Could you check a few things on this model? Use its own coordinates, in mm. Face numbers are marked on the shaded views. A direction names the side the tool comes from. Give positions to 0.01 mm unless a question says otherwise; leave off trailing zeros. Loops run counter-clockwise (first coordinate to the right, second up) from the corner with the lowest first, then second, coordinate; pieces in that order, holes last. Notation, with made-up numbers: (13.5, 50) -> (26.5, 50) arc R12 ccw to (26.5, 70) -> close; hole circle Ø1 at (55.25, 53). An arc over 180 degrees is marked (long way). Put each result on its own line as item: value.
```python
from build123d import *

# Parameters (mm, degrees)
SKETCH1_R           = 1.5
BOSS_EXTRUDE1_DEPTH = 0.85
SKETCH2_W           = 4.5
SKETCH2_H           = 18.4
BOSS_EXTRUDE2_DEPTH = 3
SKETCH3_W           = 6
SKETCH3_H           = 4.5
BOSS_EXTRUDE3_DEPTH = 3
SKETCH4_W           = 7.5
SKETCH4_H           = 5.75
BOSS_EXTRUDE4_DEPTH = 2.3
SKETCH5_W           = 20.5
SKETCH5_H           = 15.8
BOSS_EXTRUDE5_DEPTH = 7.65
SKETCH6_W           = 2.5
SKETCH6_H           = 5
BOSS_EXTRUDE6_DEPTH = 8.6
SKETCH7_W           = 20.5
SKETCH7_H           = 7
BOSS_EXTRUDE7_DEPTH = 2


with BuildPart() as part:
    # Sketch1 → Boss-Extrude1 (new, symmetric)
    with BuildSketch(Plane(origin=(0, 0, 0), x_dir=(1, 0, 0), z_dir=(0, 1, 0))):
        with BuildLine():
            Line((-15, -18), (15, -18))
            ThreePointArc((15, -18), (17.121320344, -17.121320344), (18, -15))
            Line((18, -15), (18, 15))
            ThreePointArc((18, 15), (17.121320344, 17.121320344), (15, 18))
            Line((15, 18), (-15, 18))
            ThreePointArc((-15, 18), (-17.121320344, 17.121320344), (-18, 15))
            Line((-18, 15), (-18, -15))
            ThreePointArc((-18, -15), (-17.121320344, -17.121320344), (-15, -18))
        make_face()
        with Locations(Location((-15.25, 15.25, 0), (0, 0, 270))):
            Circle(SKETCH1_R, mode=Mode.SUBTRACT)
        with Locations(Location((15.25, 15.25, 0), (0, 0, 90))):
            Circle(SKETCH1_R, mode=Mode.SUBTRACT)
        with Locations(Location((15.25, -15.25, 0), (0, 0, 270))):
            Circle(SKETCH1_R, mode=Mode.SUBTRACT)
        with Locations(Location((-15.25, -15.25, 0), (0, 0, 90))):
            Circle(SKETCH1_R, mode=Mode.SUBTRACT)
    extrude(amount=BOSS_EXTRUDE1_DEPTH, both=True)

    # Sketch2 → Boss-Extrude2 (add)
    with BuildSketch(Plane(origin=(0, 0.85, 0), x_dir=(1, 0, 0), z_dir=(0, 1, 0))):
        with Locations((-15.75, -2.4)):
            Rectangle(SKETCH2_W, SKETCH2_H)
        with Locations((15.75, -2.4)):
            Rectangle(SKETCH2_W, SKETCH2_H)
    extrude(amount=BOSS_EXTRUDE2_DEPTH)

    # Sketch3 → Boss-Extrude3 (add)
    with BuildSketch(Plane(origin=(0, 0.85, 0), x_dir=(1, 0, 0), z_dir=(0, 1, 0))):
        with Locations((-9, 15.75)):
            Rectangle(SKETCH3_W, SKETCH3_H)
        with Locations((9, 15.75)):
            Rectangle(SKETCH3_W, SKETCH3_H)
    boss_extrude3 = extrude(amount=BOSS_EXTRUDE3_DEPTH)

    # Mirror2: Boss-Extrude3 across plane
    add(boss_extrude3.mirror(Plane.ZX))

    # Sketch4 → Boss-Extrude4 (add)
    with BuildSketch(Plane(origin=(0, 0.85, 0), x_dir=(1, 0, 0), z_dir=(0, 1, 0))):
        with Locations((0, 15.525)):
            Rectangle(SKETCH4_W, SKETCH4_H)
    extrude(amount=BOSS_EXTRUDE4_DEPTH)

    # Sketch5 → Boss-Extrude5 (add)
    with BuildSketch(Plane(origin=(0, 0.85, 0), x_dir=(1, 0, 0), z_dir=(0, 1, 0))):
        with Locations((-0.95, -19.15)):
            Rectangle(SKETCH5_W, SKETCH5_H)
    extrude(amount=BOSS_EXTRUDE5_DEPTH)

    # Sketch6 → Boss-Extrude6 (add)
    with BuildSketch(Plane(origin=(0, 0.85, 0), x_dir=(1, 0, 0), z_dir=(0, 1, 0))):
        with Locations((11.3, -15.5)):
            Rectangle(SKETCH6_W, SKETCH6_H)
    extrude(amount=BOSS_EXTRUDE6_DEPTH)

    # Sketch7 → Boss-Extrude7 (add)
    with BuildSketch(Plane.XZ.offset(0.85)):
        with Locations((-0.95, 14.5)):
            Rectangle(SKETCH7_W, SKETCH7_H)
    extrude(amount=BOSS_EXTRUDE7_DEPTH)


solid = part.part
```
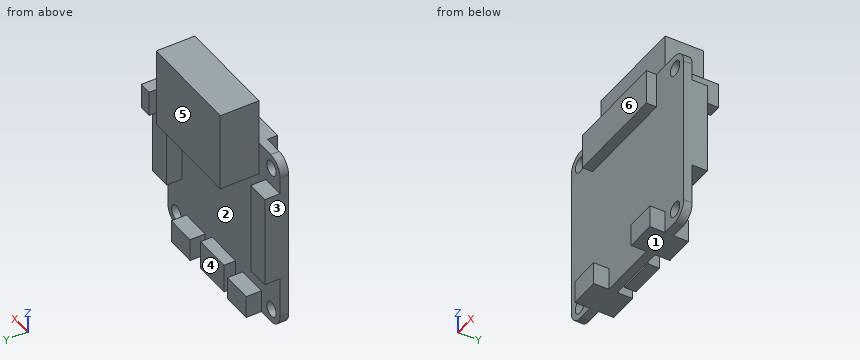
1. If we section it at A-A (y = 6.75): List the corners of the cut face in (x, z) for me.
Recorded:
outline: (-11.2, 11.25) -> (9.3, 11.25) -> (9.3, 27.05) -> (-11.2, 27.05) -> close; (10.05, 13) -> (12.55, 13) -> (12.55, 18) -> (10.05, 18) -> close
2. I need wall thicknesses on line 1 (X direction, y = 0.2, z = -15.25); line 2 (Z direction, x = 3, y = 2.25); line 3 (Z direction, x = 16, y = 0.75). Which ranges of each line are inside material? Lowest first, please.
Recorded:
line 1: x = -17.99 to -16.75, -13.75 to 13.75, 16.75 to 17.99
line 2: z = -18.4 to -12.65, 11.25 to 27.05
line 3: z = -17.83 to -16.55, -13.95 to 13.95, 16.55 to 17.83
3. If we section it at D-D (z = 12.5): List the corners of the cut face in (x, y) for me.
Recorded:
outline: (-18, -0.85) -> (-11.2, -0.85) -> (-11.2, -2.85) -> (9.3, -2.85) -> (9.3, -0.85) -> (18, -0.85) -> (18, 0.85) -> (9.3, 0.85) -> (9.3, 8.5) -> (-11.2, 8.5) -> (-11.2, 0.85) -> (-18, 0.85) -> close
4. Thinking about a two-plate mould opening in X: for the marked faces 1, 2 and 3, which applies, pulls with the +X half, pulls with the -X half, needs draft (parallel to the pull), parting line crosses it, or undercut?
Recorded:
face 1: needs draft
face 2: undercut
face 3: pulls with the -X half
5. If we section it at C-C (y = -2.25): List the corners of the cut face in (x, z) for me, then the cut area to 4 significant figures.
Recorded:
outline: (-12, -18) -> (-6, -18) -> (-6, -13.5) -> (-12, -13.5) -> close; (-11.2, 11) -> (9.3, 11) -> (9.3, 18) -> (-11.2, 18) -> close; (6, -18) -> (12, -18) -> (12, -13.5) -> (6, -13.5) -> close
area: 197.5 mm^2
6. I'm going to push flat-ended pins straight in: pin 1 (3 mm diameter, centred on x = -14, z = -1, fed in from -Y); pin 2 (3 mm diameter, centred on y = 6, z = 3.5, fed in from +X); pin 3 (3 mm diameter, centred on x = 6.5, y = 4.5, fed in from -Z); pin 4 (1.5 mm diameter, centred on y = 1.5, z = -16, fed in from -X). Where does each tip first touch, or does it pass through?
Recorded:
pin 1: stops at y = -0.85
pin 2: passes through
pin 3: stops at z = -18
pin 4: stops at x = -17.93
7. For the marked faces 4, 5 and 6, which set-ups out of +Z, -Z, +X, -X, +Y, -Y let a thin tool reach every point of the face, with its end or its side?
Recorded:
face 4: -Z, +Y
face 5: +Z, -Z, -X, +Y
face 6: +Z, +X, -X, -Y
8. If we section it at B-B (x = -6.5): List the corners of the cut face in (y, z) for me.
Recorded:
outline: (-3.85, -18) -> (3.85, -18) -> (3.85, -13.5) -> (0.85, -13.5) -> (0.85, 11.25) -> (8.5, 11.25) -> (8.5, 27.05) -> (0.85, 27.05) -> (0.85, 18) -> (-2.85, 18) -> (-2.85, 11) -> (-0.85, 11) -> (-0.85, -13.5) -> (-3.85, -13.5) -> close
